Read the model definition and answer for the solid it produces. Units are mm, in the model's axes. A direction names the side the tool comes from. Coordinates: 2 decimals unless noted, no trailing zeros. Loops run counter-clockwise (first coordinate to the right, second up) from the corner with the lowest first, then second, coordinate; pieces in that order, holes last.
Q1. Flat-ended cylindrical pins translate along their axes: P1, Ø8, axis at x = 1253, z = 474, coming from the +Y side; P2, Ø6, axis at x = 964, y = 108, coming from the -Z side; P3, Ø2, axis at x = 1099.5, z = 115, coming from the -Y side. Find the tip coordinate at first contact, or state that the pin passes through.
Q2. Section B-B (y = -208) is taken. Count the separate pieces of the cut face and the enclosed holes in it, then the cut area to 3 significant figures.
Q3. Straight lines are drawn through the part: line 1 (Z direction, x = 1355, y = 94); line 2 (Z direction, x = 521.5, y = -181.5); line 3 (Y direction, x = 357.5, z = 22). For each, find the intervals that lie inside material, in ascending order.
Q4. Section A-A (y = 80) is taken. Give the vertices of the cut face in (x, z).
Q5. Which of the six approach directions +Z, -Z, +X, -X, +Y, -Y give full straight-line access (tool end or side, diameter ignored) to faces 5 (the face through (791, 200, 45)), 6 (the face through (813, -248, 480)), 7 (the face through (799, 91, 16)), 8 (the face through (799, -232, 464)), 9 (the face through (799, -283.51, 49))?
Q6. Section C-C (x = 579) is taken. Give the vertices of the cut face in (y, z), then the cut area to 3 significant figures.
Q7. Section D-D (x = 750) is taken. Give the vertices of the cut face in (y, z).
Q8. The mould has two halves that part along X. Classify faces 1 (the face through (439, 135, 114)), 2 (the face through (979, -46, 100)), 3 (the face through (1176, -8, 114)), 4 (the face through (-16, -109, -55)): pulls with the +X half, pulls with the -X half, needs draft (parallel to the pull), parting line crosses it, or undercut.
from build123d import *

# Parameters (mm, degrees)
F1_DEPTH = 16
F3_W     = 1620
F3_H     = 484
F4_DEPTH = 16
F5_DEPTH = 14
F6_W     = 184
F6_H     = 16
F6_W_2   = 16
F6_H_2   = 464
F7_DEPTH = 1620
F9_DEPTH = 25


# Not quite as in the source:
# - a feature names something its author has since deleted; it is built from what else it names


with BuildPart() as f1:
    # F0 (on Right) → F1 (new body)
    with BuildSketch(Plane.YZ):
        Polygon((0, 480), (-300, 480), (-300, -920), (0, -920), (0, 0), (200, 0), (200, 280), align=None)
    extrude(amount=-F1_DEPTH)

    # F3 (on offset) → F4 (join)
    with BuildSketch(Plane.XY.offset(100)):
        with Locations((810, -42)):
            Rectangle(F3_W, F3_H)
        with BuildLine():
            Line((200, 140), (680, 140))
            ThreePointArc((680, 140), (687.0710678119, 137.0710678119), (690, 130))
            Line((690, 130), (690, -150))
            ThreePointArc((690, -150), (687.0710678119, -157.0710678119), (680, -160))
            Line((680, -160), (200, -160))
            ThreePointArc((200, -160), (192.9289321881, -157.0710678119), (190, -150))
            Line((190, -150), (190, 130))
            ThreePointArc((190, 130), (192.9289321881, 137.0710678119), (200, 140))
        make_face(mode=Mode.SUBTRACT)
        with BuildLine():
            Line((940, 140), (1420, 140))
            ThreePointArc((1420, 140), (1427.0710678119, 137.0710678119), (1430, 130))
            Line((1430, 130), (1430, -150))
            ThreePointArc((1430, -150), (1427.0710678119, -157.0710678119), (1420, -160))
            Line((1420, -160), (940, -160))
            ThreePointArc((940, -160), (932.9289321881, -157.0710678119), (930, -150))
            Line((930, -150), (930, 130))
            ThreePointArc((930, 130), (932.9289321881, 137.0710678119), (940, 140))
        make_face(mode=Mode.SUBTRACT)
    extrude(amount=F4_DEPTH)

    # F3 (on offset) → F5 (join)
    with BuildSketch(Plane.XY.offset(100)):
        with BuildLine():
            ThreePointArc((690, 130), (687.0710678119, 137.0710678119), (680, 140))
            Line((680, 140), (200, 140))
            ThreePointArc((200, 140), (192.9289321881, 137.0710678119), (190, 130))
            Line((190, 130), (190, -150))
            ThreePointArc((190, -150), (192.9289321881, -157.0710678119), (200, -160))
            Line((200, -160), (680, -160))
            ThreePointArc((680, -160), (687.0710678119, -157.0710678119), (690, -150))
            Line((690, -150), (690, 130))
        make_face()
        with BuildLine():
            ThreePointArc((682, -150), (681.4142135624, -151.4142135624), (680, -152))
            Line((680, -152), (200, -152))
            ThreePointArc((200, -152), (198.5857864376, -151.4142135624), (198, -150))
            Line((198, -150), (198, 130))
            ThreePointArc((198, 130), (198.5857864376, 131.4142135624), (200, 132))
            Line((200, 132), (680, 132))
            ThreePointArc((680, 132), (681.4142135624, 131.4142135624), (682, 130))
            Line((682, 130), (682, -150))
        make_face(mode=Mode.SUBTRACT)
        with BuildLine():
            ThreePointArc((1430, 130), (1427.0710678119, 137.0710678119), (1420, 140))
            Line((1420, 140), (940, 140))
            ThreePointArc((940, 140), (932.9289321881, 137.0710678119), (930, 130))
            Line((930, 130), (930, -150))
            ThreePointArc((930, -150), (932.9289321881, -157.0710678119), (940, -160))
            Line((940, -160), (1420, -160))
            ThreePointArc((1420, -160), (1427.0710678119, -157.0710678119), (1430, -150))
            Line((1430, -150), (1430, 130))
        make_face()
    extrude(amount=F5_DEPTH)

    # F6 (on face) → F7 (join)
    with BuildSketch(Plane.YZ):
        with Locations((92, 8)):
            Rectangle(F6_W, F6_H)
        Polygon((184, 100), (184, 16), (184, 0), (200, 0), (200, 100), align=None)
        with Locations((-291.5103597641, 232)):
            Rectangle(F6_W_2, F6_H_2)
        Polygon((-299.5103597641, 480), (-299.5103597641, 464), (-283.5103597641, 464), (-179.5103597641, 464), (-179.5103597641, 480), align=None)
    extrude(amount=F7_DEPTH)

    # F8 (on face) → F9 (cut)
    with BuildSketch(Plane.XY.offset(480)):
        with BuildLine():
            Line((286.6890323162, -182.5759112835), (266.6890323162, -182.5759112835))
            Line((266.6890323162, -182.5759112835), (266.6890323162, -234.4558739662))
            ThreePointArc((266.6890323162, -234.4558739662), (269.6179645043, -241.5269417781), (276.6890323162, -244.4558739662))
            ThreePointArc((276.6890323162, -244.4558739662), (283.7601001281, -241.5269417781), (286.6890323162, -234.4558739662))
            Line((286.6890323162, -234.4558739662), (286.6890323162, -182.5759112835))
        make_face()
        with BuildLine():
            Line((360.3975868225, -241.5777295828), (370.3975868225, -241.5777295828))
            ThreePointArc((370.3975868225, -241.5777295828), (377.4686546344, -238.6487973947), (380.3975868225, -231.5777295828))
            Line((380.3975868225, -231.5777295828), (380.3975868225, -171.0633635521))
            Line((380.3975868225, -171.0633635521), (350.3975868225, -171.0633635521))
            Line((350.3975868225, -171.0633635521), (350.3975868225, -231.5777295828))
            ThreePointArc((350.3975868225, -231.5777295828), (353.3265190106, -238.6487973947), (360.3975868225, -241.5777295828))
        make_face()
        with BuildLine():
            Line((173.3647221327, -231.5777295828), (173.3647221327, -174.4069010019))
            Line((173.3647221327, -174.4069010019), (133.3647221327, -174.4069010019))
            Line((133.3647221327, -174.4069010019), (133.3647221327, -231.5777295828))
            ThreePointArc((133.3647221327, -231.5777295828), (136.2936543208, -238.6487973947), (143.3647221327, -241.5777295828))
            Line((143.3647221327, -241.5777295828), (163.3647221327, -241.5777295828))
            ThreePointArc((163.3647221327, -241.5777295828), (170.4357899445, -238.6487973947), (173.3647221327, -231.5777295828))
        make_face()
        with BuildLine():
            ThreePointArc((1239.6024131775, -231.5777295828), (1242.5313453656, -238.6487973947), (1249.6024131775, -241.5777295828))
            Line((1249.6024131775, -241.5777295828), (1259.6024131775, -241.5777295828))
            ThreePointArc((1259.6024131775, -241.5777295828), (1266.6734809894, -238.6487973947), (1269.6024131775, -231.5777295828))
            Line((1269.6024131775, -231.5777295828), (1269.6024131775, -171.0633635521))
            Line((1269.6024131775, -171.0633635521), (1239.6024131775, -171.0633635521))
            Line((1239.6024131775, -171.0633635521), (1239.6024131775, -231.5777295828))
        make_face()
        with BuildLine():
            ThreePointArc((1343.3109676838, -244.4558739662), (1350.3820354957, -241.5269417781), (1353.3109676838, -234.4558739662))
            Line((1353.3109676838, -234.4558739662), (1353.3109676838, -182.5759112835))
            Line((1353.3109676838, -182.5759112835), (1333.3109676838, -182.5759112835))
            Line((1333.3109676838, -182.5759112835), (1333.3109676838, -234.4558739662))
            ThreePointArc((1333.3109676838, -234.4558739662), (1336.2398998719, -241.5269417781), (1343.3109676838, -244.4558739662))
        make_face()
        with BuildLine():
            ThreePointArc((1446.6352778673, -231.5777295828), (1449.5642100555, -238.6487973947), (1456.6352778673, -241.5777295828))
            Line((1456.6352778673, -241.5777295828), (1476.6352778673, -241.5777295828))
            ThreePointArc((1476.6352778673, -241.5777295828), (1483.7063456792, -238.6487973947), (1486.6352778673, -231.5777295828))
            Line((1486.6352778673, -231.5777295828), (1486.6352778673, -174.4069010019))
            Line((1486.6352778673, -174.4069010019), (1446.6352778673, -174.4069010019))
            Line((1446.6352778673, -174.4069010019), (1446.6352778673, -231.5777295828))
        make_face()
    extrude(amount=-F9_DEPTH, mode=Mode.SUBTRACT)


solid = f1.part
Numbers:
1. P1: stops at y = -241.56
1. P2: stops at z = 0
1. P3: stops at y = -299.51
2. separate pieces: 7
2. enclosed holes: 0
2. area: 71,400 mm2
3. line 1: z = 0 to 16, 100 to 114
3. line 2: z = 100 to 116, 464 to 480
3. line 3: y = -299.51 to -283.51, 184 to 200
4. outline: (-16, 0) - (1620, 0) - (1620, 16) - (0, 16) - (0, 100) - (198, 100) - (198, 114) - (190, 114) - (190, 116) - (0, 116) - (0, 400) - (-16, 400) - close; (682, 100) - (1620, 100) - (1620, 116) - (1430, 116) - (1430, 114) - (930, 114) - (930, 116) - (690, 116) - (690, 114) - (682, 114) - close
5. face 5: +Z, -Z, +X, -X, +Y
5. face 6: +Z, +X, -X, +Y, -Y
5. face 7: +X
5. face 8: +X, +Y
5. face 9: -Z, +X
6. outline: (-299.51, 0) - (-283.51, 0) - (-283.51, 100) - (-152, 100) - (-152, 114) - (-160, 114) - (-160, 116) - (-283.51, 116) - (-283.51, 464) - (-179.51, 464) - (-179.51, 480) - (-299.51, 480) - close; (0, 0) - (200, 0) - (200, 116) - (140, 116) - (140, 114) - (132, 114) - (132, 100) - (184, 100) - (184, 16) - (0, 16) - close
6. area: 17,000 mm2
7. outline: (-299.51, 0) - (-283.51, 0) - (-283.51, 100) - (184, 100) - (184, 16) - (0, 16) - (0, 0) - (200, 0) - (200, 116) - (-283.51, 116) - (-283.51, 464) - (-179.51, 464) - (-179.51, 480) - (-299.51, 480) - close
8. face 1: undercut
8. face 2: needs draft
8. face 3: undercut
8. face 4: pulls with the -X half
